from build123d import *

# Parameters (mm, degrees)
BOSS_EXTRUDE1_DEPTH = 7.7


with BuildPart() as part:
    # Sketch1 → Revolve1 (revolve)
    with BuildSketch(Plane.XY):
        with BuildLine():
            Line((0, 2.46), (0, 3))
            ThreePointArc((0, 3), (-0.31335038, 3.369897721), (-0.72972973, 3.121621622))
            ThreePointArc((-0.72972973, 3.121621622), (-1.119041517, 1.582340253), (-1.25, 0))
            Line((-1.25, 0), (34.1, 0))
            Line((34.1, 0), (34.1, 1.97))
            Line((34.1, 1.97), (24.85, 1.97))
            ThreePointArc((24.85, 1.97), (24.779289322, 1.999289322), (24.75, 2.07))
            Line((24.75, 2.07), (24.75, 2.36))
            ThreePointArc((24.75, 2.36), (24.720710678, 2.430710678), (24.65, 2.46))
            Line((24.65, 2.46), (0, 2.46))
        make_face()
    revolve(axis=Axis((34.1, 0, 0), (-1, 0, 0)))

    # Sketch2 → Boss-Extrude1 (add)
    with BuildSketch(Plane(origin=(22.1, 0, 0), x_dir=(0, 0, -1), z_dir=(1, 0, 0))):
        Polygon((-5.95, 3.435234102), (-5.95, -3.435234102), (0, -6.870468203), (5.95, -3.435234102), (5.95, 3.435234102), (0, 6.870468203), align=None)
    extrude(amount=-BOSS_EXTRUDE1_DEPTH)


solid = part.part
Input: part model. Units: mm. Frame: model coordinates. A direction names the side the tool comes from. Give positions to 0.01 mm unless a question says otherwise; leave off trailing zeros. Order: outer loops, then holes, each group sorted by start corner. A loop starts at its lowest first (then second) coordinate and runs counter-clockwise, first axis right, second up. Notation, with made-up numbers: (75.25, 79.25) - (93.25, 79.25) arc R12 ccw to (93.25, 99.25) - close; hole circle Ø3 at (71, -7.5). An arc over 180 degrees is marked (long way). Answer as a JSON object with one key per item and string values. Group by question number.
Q1. Cut plane C-C, the plane x = 12. Output: boundary loops of the cut face in (y, z).
Q2. First-contact query: pin 1 Ø1.5 at (x, y) = (22.5, -5) entering from -Z; pin 2 Ø1 at (x, y) = (19.5, 4.5) entering from -Z. Flat tips, straight axial feed; report the tip coordinate or a pass-through.
Q3. Cut plane B-B, the plane x = 19.5. Output: boundary loops of the cut face in (y, z).
Q4. Set-up query: faces 1 (the face through (14.4, -3, 0)), 2 (the face through (18.304, 5.129, -3.017)), 3 (the face through (22.1, -3, 0)). Return all of +Z, -Z, +X, -X, +Y, -Y with unobstructed straight access to the full face (end or side cutting, diameter ignored); none if empty.
Q5. Cut plane A-A, the plane y = 0. Output: boundary loops of the cut face in (x, z) (3 decimals).
Q6. Line query: probe 1 along X at (y, z) = (-5.25, 1.5); probe 2 along X at (y, z) = (-1.5, 2.25); probe 3 along Z at (x, y) = (26, 1.25). Output: solid intervals per line, ascending.
Results:
{
 "1": {"outline": "circle Ø4.92 at (0, 0)"},
 "2": {"pin 1": "z = -4.34", "pin 2": "z = -4.97"},
 "3": {"outline": "(-6.87, 0) - (-3.44, -5.95) - (3.44, -5.95) - (6.87, 0) - (3.44, 5.95) - (-3.44, 5.95) - close"},
 "4": {"face 1": "none", "face 2": "-Z, +X, -X, +Y", "face 3": "+X"},
 "5": {"outline": "(-0.73, -3.122) arc R0.375 ccw to (0, -3) - (0, -2.46) - (14.4, -2.46) - (14.4, -5.95) - (22.1, -5.95) - (22.1, -2.46) - (24.65, -2.46) arc R0.1 ccw to (24.75, -2.36) - (24.75, -2.07) arc R0.1 cw to (24.85, -1.97) - (34.1, -1.97) - (34.1, 1.97) - (24.85, 1.97) arc R0.1 cw to (24.75, 2.07) - (24.75, 2.36) arc R0.1 ccw to (24.65, 2.46) - (22.1, 2.46) - (22.1, 5.95) - (14.4, 5.95) - (14.4, 2.46) - (0, 2.46) - (0, 3) arc R0.375 ccw to (-0.73, 3.122) arc R9.625 ccw to start"},
 "6": {"probe 1": "14.4 to 22.1", "probe 2": "-0.86 to 0, 14.4 to 22.1", "probe 3": "-1.52 to 1.52"}
}
